Autodesk Inventor part; units mm, degrees
ref_plane "Work Plane1" through (0, 0, 5) normal (0, 0, 1) x (1, 0, 0)
ref_plane "YZ Plane" through (0, 0, 0) normal (1, 0, 0) x (0, 1, 0)
ref_plane "XZ Plane" through (0, 0, 0) normal (0, 1, 0) x (-1, 0, 0)
sketch "Sketch1" plane through (0, 0, 0) normal (0, 0, 1) x (1, 0, 0)
  circle A0 centre (0, 0) radius 25 construction
  arc A1 (0, -25) -> (0, 25) centre (0, 0) ccw
  line L0 (0, 25) -> (0, 27)
  line L1 (0, 27) -> (27, 27)
  line L2 (27, 27) -> (27, -27)
  line L3 (27, -27) -> (0, -27)
  line L4 (0, -27) -> (0, -25)
  line L5 (0, 0) -> (27, 0) construction
  dimension "d0" = 50
  dimension "d2" = 27
  dimension "d4" = 54
  dimension "d5" = 2
extrude "Extrusion1" add sketch "Sketch1" along normal blind 10
ref_plane "Work Plane1" through (0, 0, 5) normal (0, 0, 1) x (1, 0, 0)
sketch "Sketch3" plane through (0, 0, 5) normal (0, 0, 1) x (1, 0, 0)
  line L0 (27, -27) -> (27, 27)
  line L1 (27, -24) -> (21, -24)
  line L2 (0, -27) -> (27, -27)
  line L3 (21, -24) -> (21, -16.5)
  line L4 (27, -4) -> (26.4915, -4)
  arc A0 (21, -16.5) -> (26.4915, -4) centre (-3, 1.5) ccw
  line L5 (27, -4) -> (27, -24)
  point P0 (0, 0)
  dimension "d17" = 3
  dimension "d18" = 20
  dimension "d19" = 30
  dimension "d20" = 1.5
  dimension "d21" = 3
  dimension "d22" = 6
extrude "Extrusion3" cut sketch "Sketch3" along normal mid plane 6
sketch "Sketch4" plane through (0, 0, 10) normal (0, 0, 1) x (1, 0, 0)
  circle A0 centre (21, -21) radius 1.6
  point P0 (0, 0)
  dimension "d25" = 3.2
  dimension "d26" = 21
  dimension "d27" = 21
hole "Hole1" at (21, -21, 10) direction (0, 0, -1) diameter 3.2 depth 20 tip angle 118
chamfer "Chamfer2" distance 0.5 angle 45 1 edges at (27, -4, 5)
sketch "Sketch5" plane through (21, -24, 2) normal (0, 1, 0) x (1, 0, 0)
  circle A0 centre (3, -3) radius 1.6
  line L0 (11.4, -3) -> (-26.4, -3)
  line L1 (-21, 2) -> (-21, -8)
  circle A1 centre (3, -3) radius 2.75
  dimension "d38" = 3.2
  dimension "d39" = 24
  dimension "d40" = 5.5
hole "Hole2" at (24, -24, 5) direction (0, -1, 0) diameter 3.2 depth 20 tip angle 118
extrude "Extrusion4" cut sketch "Sketch5" against normal blind 3 contours L0 A1 A0 | A0 L0 A1
sketch "Sketch6" plane through (0, 0, 10) normal (0, 0, 1) x (1, 0, 0)
  line L0 (0, -27) -> (27, -27)
  line L1 (27, -27) -> (27, -29)
  line L2 (27, -29) -> (0, -29)
  line L3 (0, -29) -> (0, -27)
  line L4 (27, -27) -> (27, 27)
  line L5 (0, -25) -> (0, -27)
  line L6 (0, -27) -> (27, -27)
  point P0 (0, 0)
  dimension "d50" = 2
extrude "Extrusion5" add sketch "Sketch6" against normal blind 10
hole "Hole3" at (24, -24, 5) direction (0, -1, 0) diameter 3.2 depth 20 tip angle 118
sketch "Sketch7" plane through (0, 0, 10) normal (0, 0, 1) x (1, 0, 0)
  line L0 (27, 27) -> (0, 27)
  line L1 (0, 27) -> (27, 27)
  line L2 (27, 27) -> (27, 24)
  line L3 (27, 24) -> (0, 24)
  line L4 (0, 24) -> (0, 27)
  line L5 (27, -29) -> (27, 27)
  point P0 (0, 0)
  dimension "d60" = 3
sketch "Sketch8" plane through (0, 0, 0) normal (0, 0, -1) x (-1, 0, 0)
  circle A0 centre (-21, 21) radius 1.85
  circle A1 centre (-21, 21) radius 1.85
  circle A2 centre (-21, 21) radius 1.85
  point P0 (0, 0)
hole "Hole4" at (21, 21, 0) direction (0, 0, 1) diameter 3 depth 10
properties part number "Aufnahme_Fan_02"
Part model, mm, in its own coordinate system. A direction names the side the tool comes from. Round coordinates to 2 decimals unless told otherwise and drop trailing zeros. Loops run counter-clockwise (first coordinate to the right, second up) from the corner with the lowest first, then second, coordinate; pieces in that order, holes last. Notation, with made-up numbers: (78.5, 2.5) -> (119.5, 2.5) arc R31 cw to (119.5, 37.5) -> close; hole circle Ø2 at (81.25, 15). An arc over 180 degrees is marked (long way). Use a Markdown table: item, result.
1) Cut at C-C, the plane x = 9. List the corners of the cut face in (y, z).
The answers:
| item | result |
|---|---|
| outline | (-29, 0) -> (-23.32, 0) -> (-23.32, 10) -> (-29, 10) -> close; (23.32, 0) -> (27, 0) -> (27, 10) -> (23.32, 10) -> close |
2) Probe line 1 (X direction, y = -27.45, z = 5); line 2 (Z direction, x = 24, y = -25.85); line 3 (Z direction, x = 24, y = -28.4). List the from-to ranges inside material, lowest first. Write a range as [from, to].
The answers:
| item | result |
|---|---|
| line 1 | x = [0, 22.4], [25.6, 27] |
| line 2 | z = [0, 2.25], [7.75, 10] |
| line 3 | z = [0, 3.4], [6.6, 10] |
3) Cut at D-D, the plane z = 0.75. List the corners of the cut face in (x, y), and give its area (3 significant figures).
The answers:
| item | result |
|---|---|
| outline | (0, -29) -> (27, -29) -> (27, 27) -> (0, 27) -> (0, 25) arc R25 cw to (0, -25) -> close; hole circle Ø3.2 at (21, -21); hole circle Ø3 at (21, 21) |
| area | 515 mm2 |
4) Tool access for faces 5 (the flat face through (25, -16, 2)), 6 (the flat face through (24, -27, 3)), 7 (the flat face through (13, 27, 5)): list every direction of +Z, -Z, +X, -X, +Y, -Y with a clear straight run to the whole face (end or side of a thin tool).
The answers:
| item | result |
|---|---|
| face 5 | +X |
| face 6 | none |
| face 7 | +Z, -Z, +X, -X, +Y |
5) Cut at A-A, the plane z = 5. State how many separate pieces and enclosed holes the cut face has, and give its area (3 significant figures).
The answers:
| item | result |
|---|---|
| separate pieces | 2 |
| enclosed holes | 1 |
| area | 418 mm2 |
6) Cut at B-B, the plane y = -21. List the corners of the cut face in (x, z), and give its area (3 significant figures).
The answers:
| item | result |
|---|---|
| outline | (13.56, 0) -> (19.4, 0) -> (19.4, 10) -> (13.56, 10) -> close; (22.6, 0) -> (27, 0) -> (27, 2) -> (22.6, 2) -> close; (22.6, 8) -> (27, 8) -> (27, 10) -> (22.6, 10) -> close |
| area | 76.0 mm2 |
7) Pull direction Y, two halves, no side cores. Call faces 1 (the cylindrical face through (22.414, -28.014, 4.792)), 2 (the flat face through (21, -23, 5)), 3 (the flat face through (14, -29, 5)), 4 (the cylindrical face through (24.505, -10.478, 4.958)): pulls with the +Y half, pulls with the -Y half, needs draft (parallel to the pull), parting line crosses it, or undercut.
The answers:
| item | result |
|---|---|
| face 1 | needs draft |
| face 2 | undercut |
| face 3 | pulls with the -Y half |
| face 4 | undercut |
8) Drop flat-ended pins along their axis: pin 1 Ø2.5 at (y, z) = (-17, 5) entering from +X; pin 2 Ø2 at (x, z) = (22.5, 5) entering from -Y; pin 3 Ø2.5 at (x, z) = (24, 5) entering from -Y; pin 4 Ø3 at (y, z) = (-4, 2) entering from -X. Give the stop position or say it passes through.
The answers:
| item | result |
|---|---|
| pin 1 | stops at x = 21.54 |
| pin 2 | stops at y = -29 |
| pin 3 | stops at y = -13.89 |
| pin 4 | stops at x = 24.39 |
